Here's how the part is built. I have some questions about the finished solid (model axes, mm). Face numbers are marked on the shaded views. Coordinates: 2 decimals unless noted, no trailing zeros. Write each loop counter-clockwise with the first axis right and the second up, starting at its lowest first coordinate (ties: lowest second). Pieces come first, ordered by that corner, then holes. Notation, with made-up numbers: M 52.5,-9.75 L 94.5,-9.75 A23 cw 94.5,29.25 Z; hole C -9.75,57.5 d4. An arc over 180 degrees is marked long. Use one line per item in the form item = value. Start each with the question number.
1. Thinking about a two-plate mould opening in Z: for the marked faces 1, 2, 3 and 4, which applies, released by +Z, released by -Z, zero draft, split by the parting line, or undercut?
2. Please list where these lines run through material, in increasing order: line 1 along X through (y, z) = (0.25, 0); line 2 along X through (y, z) = (4, -1.15); line 3 along Z through (x, y) = (1.3, 4.25). Write a range as [from, to].
3. I'm going to push flat-ended pins straight in: pin 1 Ø2.5 at (x, z) = (0, 0) entering from -Y; pin 2 Ø3 at (y, z) = (-1, 2) entering from +X. Where does each tip first touch, or does it pass through?
4. I want a section at D-D, the plane z = -2.3. List the corners of the cut face in (x, y) for me.
5. I want a section at C-C, the plane z = 2.25. List the corners of the cut face in (x, y) for me.
6. I want a section at B-B, the plane y = 1. List the corners of the cut face in (x, z) for me, plus the area to 3 significant figures.
7. I want a section at A-A, the plane z = 0. List the corners of the cut face in (x, y) for me.
from build123d import *

# Parameters (mm, degrees)
SKETCH2_R           = 1.5
BOSS_EXTRUDE2_DEPTH = 7.5
CHAMFER1_SIZE       = 0.5


with BuildPart() as part:
    # Sketch2 → Boss-Extrude2 (new, symmetric)
    with BuildSketch(Plane(origin=(0, 0, 0), x_dir=(1, 0, 0), z_dir=(0, 1, 0))):
        Polygon((0, -2.886751346), (2.5, -1.443375673), (2.5, 1.443375673), (0, 2.886751346), (-2.5, 1.443375673), (-2.5, -1.443375673), align=None)
        with Locations(Location((0, 0, 0), (0, 0, 270))):
            Circle(SKETCH2_R, mode=Mode.SUBTRACT)
    extrude(amount=BOSS_EXTRUDE2_DEPTH, both=True)

    # Chamfer1
    chamfer1_edges = [part.edges().sort_by_distance(p)[0] for p in [
        (0, -7.5, -1.5),
        (0, 7.5, -1.5),
    ]]
    chamfer(chamfer1_edges, length=CHAMFER1_SIZE)

    # Sketch4 → Cut-Revolve1 (revolve, cut)
    with BuildSketch(Plane(origin=(0, 0, 0), x_dir=(0, 0, -1), z_dir=(1, 0, 0))):
        with BuildLine():
            Line((-2.886751346, 7.2), (-2.886751346, 7.5))
            Line((-2.886751346, 7.5), (-2.586751346, 7.5))
            ThreePointArc((-2.586751346, 7.5), (-2.79888338, 7.412132034), (-2.886751346, 7.2))
        make_face()
    cut_revolve1 = revolve(axis=Axis((0, 57.75, 0), (0, -1, 0)), mode=Mode.SUBTRACT)

    # Mirror1: Cut-Revolve1 across plane
    add(cut_revolve1.mirror(Plane.ZX), mode=Mode.SUBTRACT)


solid = part.part
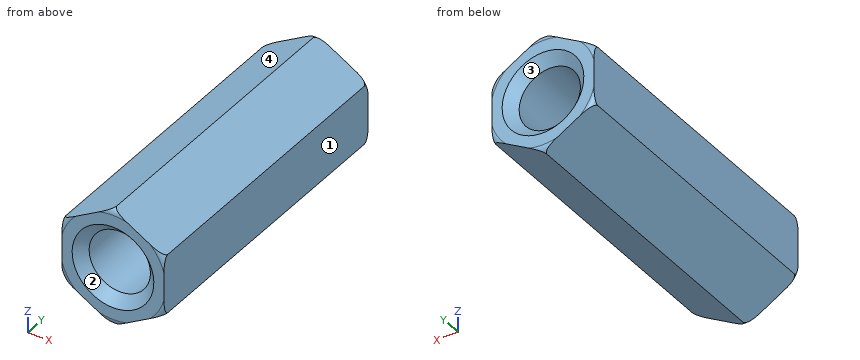
Answer list:
q1.face_1 = zero draft
q1.face_2 = undercut
q1.face_3 = undercut
q1.face_4 = released by +Z
q2.line_1 = [-2.5, -1.5], [1.5, 2.5]
q2.line_2 = [-2.5, -0.96], [0.96, 2.5]
q2.line_3 = [-2.14, -0.75], [0.75, 2.14]
q3.pin_1 = through
q3.pin_2 = 2.5
q4.outline = M -1.02,-7.5 L 1.02,-7.5 L 1.02,7.5 L -1.02,7.5 Z
q5.outline = M -1.1,-7.5 L 1.1,-7.5 L 1.1,7.5 L -1.1,7.5 Z
q6.outline = M -2.5,-1.44 L 0,-2.89 L 2.5,-1.44 L 2.5,1.44 L 0,2.89 L -2.5,1.44 Z; hole C 0,0 d3
q6.area = 14.6 mm²
q7.outline = M -2.5,-7.5 L -2,-7.5 L -1.5,-7 L -1.5,7 L -2,7.5 L -2.5,7.5 Z; M 1.5,-7 L 2,-7.5 L 2.5,-7.5 L 2.5,7.5 L 2,7.5 L 1.5,7 Z
